from build123d import *

# Parameters (mm, degrees)
F1_DEPTH = 1600


# Not quite as in the source:
# - ends of sketch curves that miss each other by under 0.0002 mm in the source are joined


with BuildPart() as f1:
    # F0 (on Front) → F1 (new body)
    with BuildSketch(Plane.XZ):
        with BuildLine():
            Line((54.9999419978, -17.7153473352), (55.0000580024, 17.7152582231))
            ThreePointArc((55.0000580024, 17.7152582231), (38.3907297006, 27.832811217), (20, 34.1586096885))
            Line((20, 34.1586096885), (20, 44.1586096885))
            Line((20, 44.1586096885), (-20, 44.1586096885))
            Line((-20, 44.1586096885), (-20, 34.1586096885))
            ThreePointArc((-20, 34.1586096885), (-38.390663502, 27.8328423177), (-54.9999419978, 17.7153473352))
            Line((-54.9999419978, 17.7153473352), (-55.0000580024, -17.7152582231))
            ThreePointArc((-55.0000580024, -17.7152582231), (-6.78258e-05, -29.8413903114), (54.9999419978, -17.7153473352))
        make_face()
    extrude(amount=F1_DEPTH)


solid = f1.part
Geometry check sheet. Reference: the model listing, model coordinates, mm. Round coordinates to 2 decimals unless told otherwise and drop trailing zeros. Order: outer loops, then holes, each group sorted by start corner. A loop starts at its lowest first (then second) coordinate and runs counter-clockwise, first axis right, second up. Notation, with made-up numbers: (64, 89.5) -> (118, 89.5) arc R15 cw to (118, 117.5) -> close; hole circle Ø5 at (61, 78.5). An arc over 180 degrees is marked (long way). Use one line per item in the form item = value.
1. Cross-section at A-A, the plane y = -1157.5. Enter the section's corners in (x, z).
Working result:
outline = (-55, -17.72) arc R130.79 ccw to (55, -17.72) -> (55, 17.72) arc R90.28 ccw to (20, 34.16) -> (20, 44.16) -> (-20, 44.16) -> (-20, 34.16) arc R90.28 ccw to (-55, 17.72) -> close
2. Go/stop test with flat-tipped pins: pin 1 (1.5 mm diameter, centred on x = -30.5, y = -1242.5, fed in from -Z); pin 2 (8 mm diameter, centred on y = -628, z = 40, fed in from -X); pin 3 (6 mm diameter, centred on x = -13.5, y = -1341.5, fed in from -Z). Record where each tip stops, or that it passes through.
Working result:
pin_1 = -26.41
pin_2 = -20
pin_3 = -29.42
3. Scan lines: line 1 along Z through (x, y) = (-27, -1434.5); line 2 along Z through (x, y) = (0, -657); line 3 along X through (y, z) = (-866, 23.5). Record each from-to range of solid material in increasing order. Write a range as from..to.
Working result:
line_1 = -27.02..32.27
line_2 = -29.84..44.16
line_3 = -46.51..46.51
